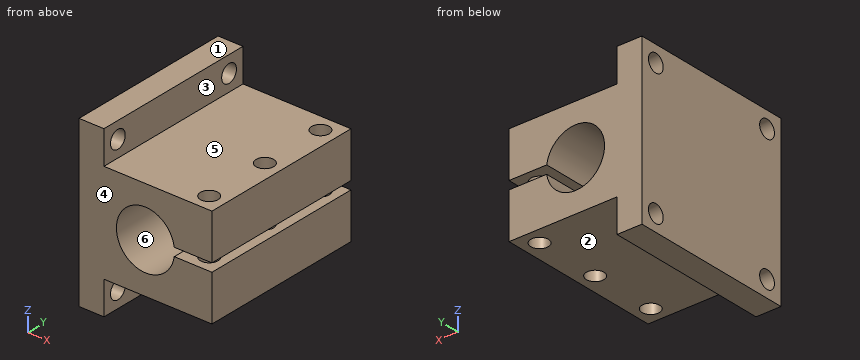
```python
from build123d import *

# Parameters (mm, degrees)
SKETCH1_W                   = 50.8
SKETCH1_H                   = 63.5
BOSS_EXTRUDE1_DEPTH         = 63.5
SKETCH2_R                   = 11.1125
CUT_EXTRUDE1_DEPTH          = 76.402072253
SKETCH3_W                   = 41.275
SKETCH3_H                   = 12.7
CUT_EXTRUDE2_DEPTH          = 76.402072253
F_1_4_CLEARANCE_HOLE1_D     = 6.7564
F_1_4_CLEARANCE_HOLE1_DEPTH = 9.652
F_1_4_CLEARANCE_HOLE1_TIP   = 2.029827343
SKETCH6_W                   = 3.175
SKETCH6_H                   = 63.5
CUT_EXTRUDE3_DEPTH          = 24.13
F_1_4_CLEARANCE_HOLE2_D     = 6.7564


with BuildPart() as part:
    # Sketch1 → Boss-Extrude1 (new body)
    with BuildSketch(Plane(origin=(0, 0, 0), x_dir=(1, 0, 0), z_dir=(0, 1, 0))):
        Rectangle(SKETCH1_W, SKETCH1_H)
    extrude(amount=BOSS_EXTRUDE1_DEPTH)

    # Sketch2 → Cut-Extrude1 (cut, through all)
    with BuildSketch(Plane(origin=(0, 63.5, 0), x_dir=(1, 0, 0), z_dir=(0, 1, 0))):
        with Locations(Location((0, 0, 0), (0, 0, 270))):
            Circle(SKETCH2_R)
    extrude(amount=-CUT_EXTRUDE1_DEPTH, mode=Mode.SUBTRACT)

    # Sketch3 → Cut-Extrude2 (cut, through all)
    with BuildSketch(Plane(origin=(0, 63.5, 0), x_dir=(1, 0, 0), z_dir=(0, 1, 0))):
        with Locations((4.7625, 25.4)):
            Rectangle(SKETCH3_W, SKETCH3_H)
        with Locations((4.7625, -25.4)):
            Rectangle(SKETCH3_W, SKETCH3_H)
    extrude(amount=-CUT_EXTRUDE2_DEPTH, mode=Mode.SUBTRACT)

    # 1/4 Clearance Hole1
    with Locations(Plane(origin=(-15.875, 0, 0), x_dir=(0, 0, -1), z_dir=(1, 0, 0))):
        with Locations((-25.4, 57.15), (25.4, 6.35), (-25.4, 6.35), (25.4, 57.15)):
            Hole(F_1_4_CLEARANCE_HOLE1_D / 2, depth=F_1_4_CLEARANCE_HOLE1_DEPTH)
            with Locations((0, 0, -(F_1_4_CLEARANCE_HOLE1_DEPTH + F_1_4_CLEARANCE_HOLE1_TIP / 2))):  # 118° drill point
                Cone(0, F_1_4_CLEARANCE_HOLE1_D / 2, F_1_4_CLEARANCE_HOLE1_TIP, mode=Mode.SUBTRACT)

    # Sketch6 → Cut-Extrude3 (cut)
    with BuildSketch(Plane(origin=(25.4, 0, 0), x_dir=(0, 0, -1), z_dir=(1, 0, 0))):
        with Locations((0, 31.75)):
            Rectangle(SKETCH6_W, SKETCH6_H)
    extrude(amount=-CUT_EXTRUDE3_DEPTH, mode=Mode.SUBTRACT)

    # 1/4 Clearance Hole2 (through all)
    with Locations(Plane.XY.offset(19.05)):
        with Locations((19.05, 57.15), (19.05, 31.75), (19.05, 6.35)):
            Hole(F_1_4_CLEARANCE_HOLE2_D / 2)


solid = part.part
```
Model file for the job. Use its own axes, mm. Face numbers are marked on the shaded views. A direction names the side the tool comes from. Coordinates: 2 decimals unless noted, no trailing zeros. Write each loop counter-clockwise with the first axis right and the second up, starting at its lowest first coordinate (ties: lowest second). Pieces come first, ordered by that corner, then holes. Notation, with made-up numbers: (49.5, 54) - (55.5, 54) arc R14 ccw to (55.5, 61) - close; hole circle Ø2 at (58.25, 62.5). An arc over 180 degrees is marked (long way). One line per item, written item: value. Start each with the question number.
1. Flat gauge pins, fed straight in: pin 1 (3 mm diameter, centred on x = 6, y = 38.5, fed in from +Z); pin 2 (5 mm diameter, centred on x = -1, y = 27.5, fed in from -Z). Where does each tip first touch, or does it go through?
2. Mould opens along Z. For the marked faces 4, 5 and 6 say: released by +Z, released by -Z, zero draft, split by the parting line, or undercut.
3. Probe line 1 (Y direction, x = -22.5, z = 25.4); line 2 (Y direction, x = 19.05, z = -10.5); line 3 (Z direction, x = 19, y = 49). List the from-to ranges inside material, lowest first. Write a range as from..to.
4. Slice it at A-A (x = 0). Write the cut outline in (y, z), plus the area to 3 significant figures.
5. Tool access for the marked faces 1, 2 and 3: list every direction of +Z, -Z, +X, -X, +Y, -Y with a clear straight run to the whole face (end or side of a thin tool).
6. Slice it at B-B (z = 25.4). Write the cut outline in (x, y) (3 decimals).
7. Slice it at C-C (y = 31.75). Count the separate pieces of the cut face and the enclosed holes in it, plus the area to 3 significant figures.
Answers below:
1. pin 1: stops at z = 19.05
1. pin 2: stops at z = -19.05
2. face 4: zero draft
2. face 5: released by +Z
2. face 6: undercut
3. line 1: y = 0..2.97, 9.73..53.77, 60.53..63.5
3. line 2: y = 0..2.97, 9.73..28.37, 35.13..53.77, 60.53..63.5
3. line 3: z = -19.05..-1.59, 1.59..19.05
4. outline: (0, -19.05) - (63.5, -19.05) - (63.5, -11.11) - (0, -11.11) - close; (0, 11.11) - (63.5, 11.11) - (63.5, 19.05) - (0, 19.05) - close
4. area: 1,010 mm^2
5. face 1: +Z, +X, -X, +Y, -Y
5. face 2: -Z, +X, +Y, -Y
5. face 3: +Z, +X, +Y, -Y
6. outline: (-25.4, 0) - (-15.875, 0) - (-15.875, 2.972) - (-25.4, 2.972) - close; (-25.4, 9.728) - (-15.875, 9.728) - (-15.875, 53.772) - (-25.4, 53.772) - close; (-25.4, 60.528) - (-15.875, 60.528) - (-15.875, 63.5) - (-25.4, 63.5) - close
7. separate pieces: 3
7. enclosed holes: 0
7. area: 1,510 mm^2
